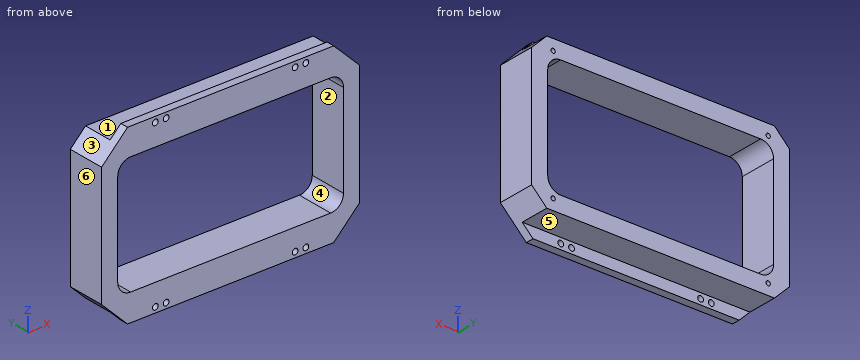
from build123d import *

# Parameters (mm, degrees)
SKETCH1_W                   = 304.8
SKETCH1_H                   = 177.8
BOSS_EXTRUDE1_DEPTH         = 44.45
CHAMFER1_SIZE               = 17.9578
CUT_EXTRUDE1_DEPTH          = 45.45
F_1_4_20_TAPPED_HOLE1_D     = 5.1054
F_1_4_20_TAPPED_HOLE1_DEPTH = 19.05
F_1_4_20_TAPPED_HOLE1_TIP   = 1.533816902
BOSS_EXTRUDE2_DEPTH         = 9.525
F_1_4_CLEARANCE_HOLE1_D     = 6.7564
FILLET2_R                   = 15.24


with BuildPart() as part:
    # Sketch1 → Boss-Extrude1 (new body)
    with BuildSketch(Plane(origin=(0, 0, 0), x_dir=(1, 0, 0), z_dir=(0, 1, 0))):
        Rectangle(SKETCH1_W, SKETCH1_H)
    extrude(amount=BOSS_EXTRUDE1_DEPTH)

    # Chamfer1
    chamfer1_edges = [part.edges().sort_by_distance(p)[0] for p in [
        (-152.4, 22.225, -88.9),
        (152.4, 22.225, -88.9),
        (152.4, 22.225, 88.9),
        (-152.4, 22.225, 88.9),
    ]]
    chamfer(chamfer1_edges, length=CHAMFER1_SIZE)

    # Sketch3 → Cut-Extrude1 (cut, through all)
    with BuildSketch(Plane(origin=(0, 44.45, 0), x_dir=(1, 0, 0), z_dir=(0, 1, 0))):
        Polygon((133.35, 63.051431637), (126.551431637, 69.85), (-126.551431637, 69.85), (-133.35, 63.051431637), (-133.35, -63.051431637), (-126.551431637, -69.85), (126.551431637, -69.85), (133.35, -63.051431637), align=None)
        Polygon((-133.35, 63.051431637), (-126.551431637, 69.85), (-133.35, 69.85), align=None)
        Polygon((133.35, 69.85), (126.551431637, 69.85), (133.35, 63.051431637), align=None)
        Polygon((-126.551431637, -69.85), (-133.35, -63.051431637), (-133.35, -69.85), align=None)
        Polygon((133.35, -69.85), (133.35, -63.051431637), (126.551431637, -69.85), align=None)
    extrude(amount=-CUT_EXTRUDE1_DEPTH, mode=Mode.SUBTRACT)

    # 1/4-20 Tapped Hole1
    with Locations(Plane(origin=(0, 44.45, 0), x_dir=(1, 0, 0), z_dir=(0, 1, 0))):
        with Locations((-127, 76.2), (127, 76.2), (127, -76.2), (-127, -76.2)):
            Hole(F_1_4_20_TAPPED_HOLE1_D / 2, depth=F_1_4_20_TAPPED_HOLE1_DEPTH)
            with Locations((0, 0, -(F_1_4_20_TAPPED_HOLE1_DEPTH + F_1_4_20_TAPPED_HOLE1_TIP / 2))):  # 118° drill point
                Cone(0, F_1_4_20_TAPPED_HOLE1_D / 2, F_1_4_20_TAPPED_HOLE1_TIP, mode=Mode.SUBTRACT)

    # Sketch6 → Boss-Extrude2 (add)
    with BuildSketch(Plane.XZ):
        Polygon((121.7422, 101.6), (134.4422, 88.9), (-134.4422, 88.9), (-121.7422, 101.6), align=None)
    boss_extrude2 = extrude(amount=-BOSS_EXTRUDE2_DEPTH)

    # 1/4 Clearance Hole1 (through all)
    with Locations(Plane(origin=(0, 9.525, 0), x_dir=(1, 0, 0), z_dir=(0, 1, 0))):
        with Locations((-88.9, -95.25), (88.9, -95.25), (-76.2, -95.25), (76.2, -95.25)):
            f_1_4_clearance_hole1 = Hole(F_1_4_CLEARANCE_HOLE1_D / 2)

    # Mirror1: Boss-Extrude2, 1/4 Clearance Hole1 across plane
    add(boss_extrude2.mirror(Plane.XY))
    add(f_1_4_clearance_hole1.mirror(Plane.XY), mode=Mode.SUBTRACT)

    # Fillet2
    fillet2_edges = [part.edges().sort_by_distance(p)[0] for p in [
        (133.35, 22.225, -69.85),
        (133.35, 22.225, 69.85),
        (-133.35, 22.225, 69.85),
        (-133.35, 22.225, -69.85),
    ]]
    fillet(fillet2_edges, radius=FILLET2_R)


solid = part.part
Geometry check sheet. Reference: the model listing, model coordinates, mm. Face numbers are marked on the shaded views. A direction names the side the tool comes from. Round coordinates to 2 decimals unless told otherwise and drop trailing zeros. Loops run counter-clockwise (first coordinate to the right, second up) from the corner with the lowest first, then second, coordinate; pieces in that order, holes last.
Item 1: Access from +Z, -Z, +X, -X, +Y, -Y to the whole of each face (thin tool, end or side, straight path). Record for the marked faces 1, 2 and 3.
Item 2: Thickness scan on line 1 (X direction, y = 29, z = 47.5); line 2 (Z direction, x = -16, y = 39); line 3 (X direction, y = 7.5, z = 95.25). Record the ranges inside material, lowest first.
Item 3: Cross-section at B-B on z = 14.5. Record the boundary of the cut face in (x, y), then the cut area to 3 significant figures.
Item 4: Mould release check, pull along X, two halves, no side actions. Record for the marked faces 4, 5 and 6: pulls with the +X half, pulls with the -X half, needs draft (parallel to the pull), parting line crosses it, or undercut.
Item 5: Cross-section at A-A on x = 31. Record the boundary of the cut face in (y, z) (3 decimals), then the cut area to 3 significant figures.
Item 6: Cross-section at C-C on y = 14.5. Record the boundary of the cut face in (x, z), then the cut area to 3 significant figures.
Item 7: Cross-section at D-D on x = 88.9. Record the boundary of the cut face in (y, z) (3 decimals), then the cut area to 3 significant figures.
Item 8: Gauge pin test, flat ends, axial feed: pin 1 (10 mm diameter, centred on x = -104.5, y = 16.5, fed in from +Z); pin 2 (8 mm diameter, centred on x = -88.9, z = 95.25, fed in from -Y); pin 3 (8 mm diameter, centred on x = -76.2, z = -95.25, fed in from +Y) (3 decimals); pin 4 (6 mm diameter, centred on x = 76.2, z = 95.25, fed in from +Y). Record the tip position at first contact, or that the pin passes through.
Answer sheet:
1. face 1: +Z, +X, -X, +Y
1. face 2: +Y, -Y
1. face 3: +Z, -X, +Y, -Y
2. line 1: x = -152.4 to -133.35, 133.35 to 152.4
2. line 2: z = -88.9 to -69.85, 69.85 to 88.9
2. line 3: x = -128.09 to -92.28, -85.52 to -79.58, -72.82 to 72.82, 79.58 to 85.52, 92.28 to 128.09
3. outline: (-152.4, 0) - (-133.35, 0) - (-133.35, 44.45) - (-152.4, 44.45) - close; (133.35, 0) - (152.4, 0) - (152.4, 44.45) - (133.35, 44.45) - close
3. area: 1,690 mm2
4. face 4: undercut
4. face 5: needs draft
4. face 6: pulls with the -X half
5. outline: (0, -101.6) - (9.525, -101.6) - (9.525, -88.9) - (44.45, -88.9) - (44.45, -69.85) - (0, -69.85) - close; (0, 69.85) - (44.45, 69.85) - (44.45, 88.9) - (9.525, 88.9) - (9.525, 101.6) - (0, 101.6) - close
5. area: 1,940 mm2
6. outline: (-152.4, -70.94) - (-134.44, -88.9) - (134.44, -88.9) - (152.4, -70.94) - (152.4, 70.94) - (134.44, 88.9) - (-134.44, 88.9) - (-152.4, 70.94) - close; hole (-133.35, -54.61) arc R15.24 ccw to (-118.11, -69.85) - (118.11, -69.85) arc R15.24 ccw to (133.35, -54.61) - (133.35, 54.61) arc R15.24 ccw to (118.11, 69.85) - (-118.11, 69.85) arc R15.24 ccw to (-133.35, 54.61) - close
6. area: 16,500 mm2
7. outline: (0, -101.6) - (9.525, -101.6) - (9.525, -98.628) - (0, -98.628) - close; (0, -91.872) - (9.525, -91.872) - (9.525, -88.9) - (44.45, -88.9) - (44.45, -69.85) - (0, -69.85) - close; (0, 69.85) - (44.45, 69.85) - (44.45, 88.9) - (9.525, 88.9) - (9.525, 91.872) - (0, 91.872) - close; (0, 98.628) - (9.525, 98.628) - (9.525, 101.6) - (0, 101.6) - close
7. area: 1,810 mm2
8. pin 1: stops at z = 88.9
8. pin 2: stops at y = 0
8. pin 3: stops at y = 9.525
8. pin 4: passes through
